```python
from build123d import *

# Parameters (mm, degrees)
SKETCH1_W           = 112.7
SKETCH1_H           = 100
BOSS_EXTRUDE1_DEPTH = 6.35
SKETCH2_W           = 6.35
SKETCH2_H           = 12.7
CUT_EXTRUDE1_DEPTH  = 7.35
CIRPATTERN1_COUNT   = 2
SKETCH5_W           = 12.7
SKETCH5_H           = 6.35
BOSS_EXTRUDE2_DEPTH = 6.35
SKETCH6_W           = 19.05
SKETCH6_H           = 6.35
BOSS_EXTRUDE3_DEPTH = 59.05
SKETCH7_W           = 12.7
SKETCH7_H           = 6.35
BOSS_EXTRUDE4_DEPTH = 10


with BuildPart() as part:
    # Sketch1 → Boss-Extrude1 (new body)
    with BuildSketch(Plane(origin=(0, 0, 0), x_dir=(1, 0, 0), z_dir=(0, 1, 0))):
        Rectangle(SKETCH1_W, SKETCH1_H)
    extrude(amount=BOSS_EXTRUDE1_DEPTH)

    # Sketch2 → Cut-Extrude1 (cut, through all)
    with BuildSketch(Plane(origin=(0, 6.35, 0), x_dir=(1, 0, 0), z_dir=(0, 1, 0))):
        with Locations((53.175, 0)):
            Rectangle(SKETCH2_W, SKETCH2_H)
    cut_extrude1 = extrude(amount=-CUT_EXTRUDE1_DEPTH, mode=Mode.SUBTRACT)

    # CirPattern1: Cut-Extrude1 ×2 about axis
    cirpattern1_axis = Axis((0, 0, 0), (0, 1, 0))
    for i in range(1, CIRPATTERN1_COUNT):
        add(cut_extrude1.rotate(cirpattern1_axis, i * 360 / CIRPATTERN1_COUNT), mode=Mode.SUBTRACT)

    # Sketch5 → Boss-Extrude2 (add)
    with BuildSketch(Plane.XY.offset(50)):
        with Locations((0, 3.175)):
            Rectangle(SKETCH5_W, SKETCH5_H)
    extrude(amount=BOSS_EXTRUDE2_DEPTH)

    # Sketch6 → Boss-Extrude3 (add)
    with BuildSketch(Plane.XY.offset(50)):
        with Locations((-46.825, 3.175)):
            Rectangle(SKETCH6_W, SKETCH6_H)
    boss_extrude3 = extrude(amount=BOSS_EXTRUDE3_DEPTH)

    # Mirror1: Boss-Extrude3 across plane
    add(boss_extrude3.mirror(Plane(origin=(0, 0, 0), x_dir=(0, 0, 1), z_dir=(1, 0, 0))))

    # Sketch7 → Boss-Extrude4 (add)
    with BuildSketch(Plane(origin=(0, 0, -50), x_dir=(-1, 0, 0), z_dir=(0, 0, -1))):
        with Locations((0, 3.175)):
            Rectangle(SKETCH7_W, SKETCH7_H)
    extrude(amount=BOSS_EXTRUDE4_DEPTH)


solid = part.part
```
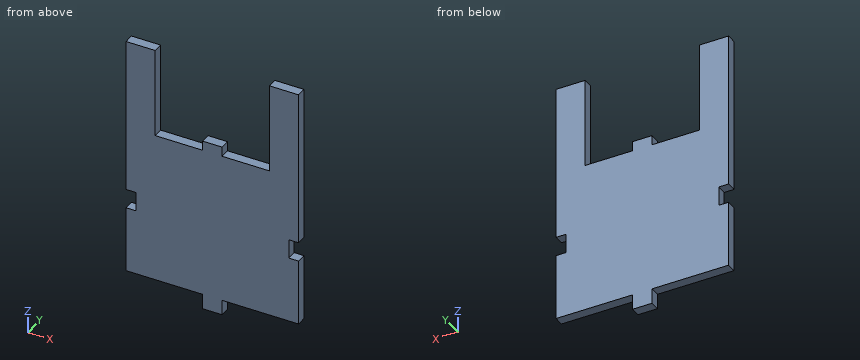
For this review, take the finished solid that the model builds, in its own axes (mm). Round coordinates to 2 decimals unless told otherwise and drop trailing zeros. Write each loop counter-clockwise with the first axis right and the second up, starting at its lowest first coordinate (ties: lowest second). Pieces come first, ordered by that corner, then holes.
1) Take a section at B-B on y = 4.5. Give the boundary of the cut face in (x, z).
Answer below:
outline: (-56.35, -50) - (-6.35, -50) - (-6.35, -60) - (6.35, -60) - (6.35, -50) - (56.35, -50) - (56.35, -6.35) - (50, -6.35) - (50, 6.35) - (56.35, 6.35) - (56.35, 109.05) - (37.3, 109.05) - (37.3, 50) - (6.35, 50) - (6.35, 56.35) - (-6.35, 56.35) - (-6.35, 50) - (-37.3, 50) - (-37.3, 109.05) - (-56.35, 109.05) - (-56.35, 6.35) - (-50, 6.35) - (-50, -6.35) - (-56.35, -6.35) - close
2) Insertion check: pin 1 Ø1.9 at (x, y) = (-15.5, 2) entering from +Z; pin 2 Ø1.9 at (y, z) = (3.5, -54) entering from +X; pin 3 Ø3 at (x, y) = (-2, 2) entering from +Z. Each pin has a flat end and moves straight along its axis. Give the tip position at first contact, or say it passes through.
Answer below:
pin 1: stops at z = 50
pin 2: stops at x = 6.35
pin 3: stops at z = 56.35
3) Take a section at C-C on x = -3. Give the boundary of the cut face in (y, z), then the cut area to 3 significant figures.
Answer below:
outline: (0, -60) - (6.35, -60) - (6.35, 56.35) - (0, 56.35) - close
area: 739 mm2
4) Take a section at A-A on z = 78.5. Give the boundary of the cut face in (x, y), then the cut area to 3 significant figures.
Answer below:
outline: (-56.35, 0) - (-37.3, 0) - (-37.3, 6.35) - (-56.35, 6.35) - close; (37.3, 0) - (56.35, 0) - (56.35, 6.35) - (37.3, 6.35) - close
area: 242 mm2
5) Take a section at D-D on x = -47.5. Give the boundary of the cut face in (y, z).
Answer below:
outline: (0, -50) - (6.35, -50) - (6.35, 109.05) - (0, 109.05) - close
6) For line 1 along X through (y, z) = (3.5, 76); line 2 along Z through (x, y) = (26, 5.75); line 3 along Z through (x, y) = (6, 6), list the stretches that pass through material, from the lowest coordinate up.
Answer below:
line 1: x = -56.35 to -37.3, 37.3 to 56.35
line 2: z = -50 to 50
line 3: z = -60 to 56.35
